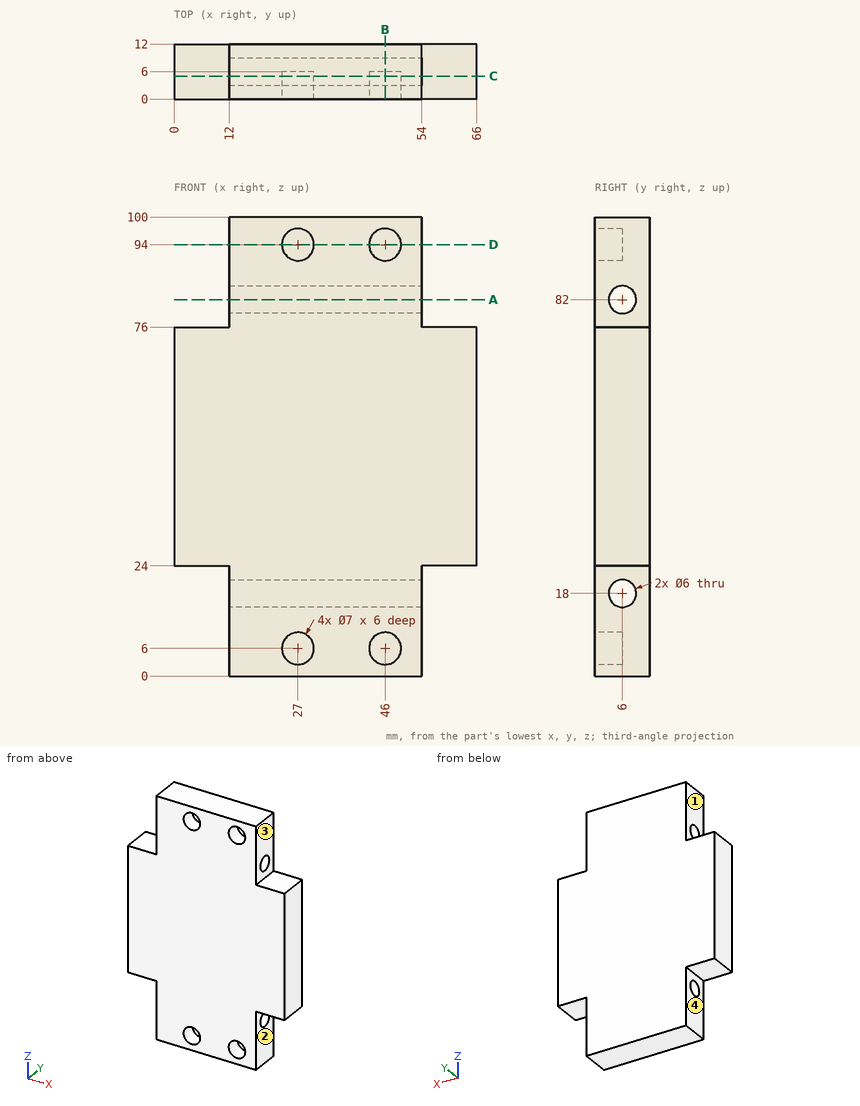
Input: dimensioned drawing with shaded views. Units: mm. Origin: part minimum x, y, z. A direction names the side the tool comes from. Round coordinates to 2 decimals unless told otherwise and drop trailing zeros. Write each loop counter-clockwise with the first axis right and the second up, starting at its lowest first coordinate (ties: lowest second). Pieces come first, ordered by that corner, then holes. Notation, with made-up numbers: (47, 58) -> (51, 58) arc R22 ccw to (51, 86) -> close; hole circle Ø1 at (37.5, -18.5). An arc over 180 degrees is marked (long way). Use CSV: the item, a comma, the result in double quotes. Start each with the question number.
Q1. Reachability of the marked faces 1, 2, 3 and 4 from +Z, -Z, +X, -X, +Y, -Y: full face, straight path, thin tool, end or side. Return the list, or none.
Q2. Section A-A (z = 82). Return loops of the section in (x, y).
Q3. Section C-C (y = 5). Return loops of the section in (x, z), plus the area to 3 significant figures.
Q4. Section D-D (z = 94). Return loops of the section in (x, y), plus the area to 3 significant figures.
Q5. First-contact query: pin 1 Ø3.5 at (x, y) = (57.5, 6) entering from -Z; pin 2 Ø3.5 at (y, z) = (7.5, 93) entering from -X; pin 3 Ø1.5 at (x, y) = (57, 5) entering from +Z. Flat tips, straight axial feed; report the tip coordinate or a pass-through.
Q6. Section B-B (x = 46). Return loops of the section in (y, z), plus the area to 3 significant figures.
Q7. Line query: L1, parallel to Z at x = 48, y = 2.75; L2, parallel to Z at x = 28, y = 5; L3, parallel to Z at x = 46, y = 4.3. Output: solid intervals per line, ascending.
Result sheet:
1,face 1,"+Z, -X, +Y, -Y"
1,face 2,"-Z, +X, +Y, -Y"
1,face 3,"+Z, +X, +Y, -Y"
1,face 4,"-Z, -X, +Y, -Y"
2,outline,"(12, 0) -> (54, 0) -> (54, 3) -> (12, 3) -> close; (12, 9) -> (54, 9) -> (54, 12) -> (12, 12) -> close"
3,outline,"(0, 24) -> (12, 24) -> (12, 20.83) -> (54, 20.83) -> (54, 24) -> (66, 24) -> (66, 76) -> (54, 76) -> (54, 79.17) -> (12, 79.17) -> (12, 76) -> (0, 76) -> close; (12, 0) -> (54, 0) -> (54, 15.17) -> (12, 15.17) -> close; (12, 84.83) -> (54, 84.83) -> (54, 100) -> (12, 100) -> close; hole circle Ø7 at (27, 6); hole circle Ø7 at (27, 94); hole circle Ø7 at (46, 6); hole circle Ø7 at (46, 94)"
3,area,"4,820 mm²"
4,outline,"(12, 0) -> (23.5, 0) -> (23.5, 6) -> (30.5, 6) -> (30.5, 0) -> (42.5, 0) -> (42.5, 6) -> (49.5, 6) -> (49.5, 0) -> (54, 0) -> (54, 12) -> (12, 12) -> close"
4,area,"420 mm²"
5,pin 1,"z = 24"
5,pin 2,"x = 12"
5,pin 3,"z = 76"
6,outline,"(0, 0) -> (12, 0) -> (12, 100) -> (0, 100) -> (0, 97.5) -> (6, 97.5) -> (6, 90.5) -> (0, 90.5) -> (0, 9.5) -> (6, 9.5) -> (6, 2.5) -> (0, 2.5) -> close; hole circle Ø6 at (6, 18); hole circle Ø6 at (6, 82)"
6,area,"1,060 mm²"
7,L1,"0 to 3.13, 8.87 to 91.13, 96.87 to 100"
7,L2,"0 to 2.65, 9.35 to 15.17, 20.83 to 79.17, 84.83 to 90.65, 97.35 to 100"
7,L3,"0 to 2.5, 9.5 to 15.53, 20.47 to 79.53, 84.47 to 90.5, 97.5 to 100"
